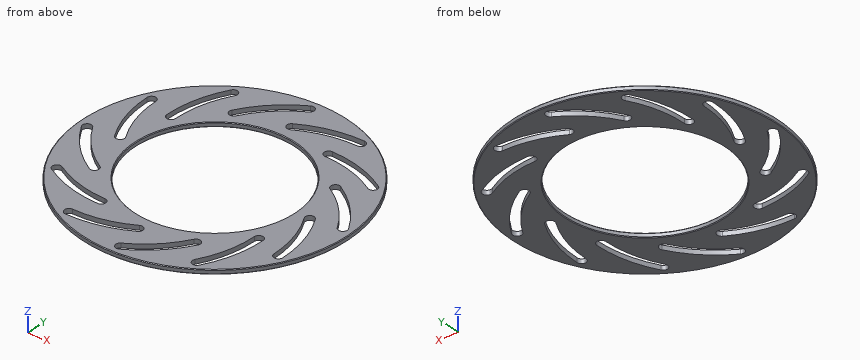
from build123d import *

# Parameters (mm, degrees)
SKETCH1_R           = 60
SKETCH1_R_2         = 36
BOSS_EXTRUDE1_DEPTH = 2
CUT_EXTRUDE1_DEPTH  = 85.876380696
CIRPATTERN1_COUNT   = 12
CHAMFER1_SIZE       = 0.3


with BuildPart() as part:
    # Sketch1 → Boss-Extrude1 (new body)
    with BuildSketch(Plane.XY):
        Circle(SKETCH1_R)
        Circle(SKETCH1_R_2, mode=Mode.SUBTRACT)
    extrude(amount=BOSS_EXTRUDE1_DEPTH)

    # Sketch2 → Cut-Extrude1 (cut, through all)
    with BuildSketch(Plane.XY.offset(2)):
        with BuildLine():
            ThreePointArc((25.722326885, 51.193712683), (11.890599802, 49.519139452), (-1, 44.232050808))
            ThreePointArc((-1, 44.232050808), (-1.732050808, 41.5), (1, 40.767949192))
            ThreePointArc((1, 40.767949192), (12.899015202, 45.64833871), (25.666763279, 47.194098616))
            ThreePointArc((25.666763279, 47.194098616), (27.694352115, 49.166123846), (25.722326885, 51.193712683))
        make_face()
    cut_extrude1 = extrude(amount=-CUT_EXTRUDE1_DEPTH, mode=Mode.SUBTRACT)

    # CirPattern1: Cut-Extrude1 ×12 about axis
    cirpattern1_axis = Axis((0, 0, 0), (0, 0, 1))
    for i in range(1, CIRPATTERN1_COUNT):
        add(cut_extrude1.rotate(cirpattern1_axis, i * 360 / CIRPATTERN1_COUNT), mode=Mode.SUBTRACT)

    # Chamfer1
    chamfer1_edges = [part.edges().sort_by_distance(p)[0] for p in [
        (-60, 0, 0),
        (-60, 0, 2),
        (-36, 0, 0),
        (-36, 0, 2),
    ]]
    chamfer(chamfer1_edges, length=CHAMFER1_SIZE)


solid = part.part
Check sheet for the modelled part. Datum: model origin and axes. Units: mm. Round coordinates to 2 decimals unless told otherwise and drop trailing zeros.
(1) Scan lines: probe 1 along Y at (x, z) = (0, 0.9); probe 2 along Y at (x, z) = (27, 1.6); probe 3 along X at (y, z) = (15.5, 1.8). Record each from-to range of solid material in increasing order.
(2) Cross-section at A-A, the plane x = 14. State how many separate pieces and enclosed holes the cut face has, and give its area (3 significant figures).
(3) Go/stop test with a flat-tipped pin: P1, Ø1, axis at x = 18.5, z = 1.5, coming from the -Y side. Record where the tip stops, or that it passes through.
Check sheet entries:
1. probe 1: y = -60 to -44.79, -40.5 to -36, 36 to 40.5, 44.79 to 60
1. probe 2: y = -53.58 to -23.81, 23.81 to 34.46, 38.49 to 47.68, 50.71 to 53.58
1. probe 3: x = -57.86 to -50.32, -46.25 to -32.6, 32.6 to 41.7, 47.78 to 57.86
2. separate pieces: 4
2. enclosed holes: 0
2. area: 80.6 mm2
3. P1: stops at y = -57.24
